The figure shows three views and two pictorial views of one solid part (mm, origin at its lowest corner). Answer the questions. A direction names the side the tool comes from. Give positions to 0.01 mm unless a question says otherwise; leave off trailing zeros. Write each loop counter-clockwise with the first axis right and the second up, starting at its lowest first coordinate (ties: lowest second). Pieces come first, ordered by that corner, then holes. Notation, with made-up numbers: M 44.5,41 L 69.5,41 A30 cw 69.5,63 Z; hole C -16.5,-28 d11. An arc over 180 degrees is marked long. Return JSON: item names as keys, results as strings.
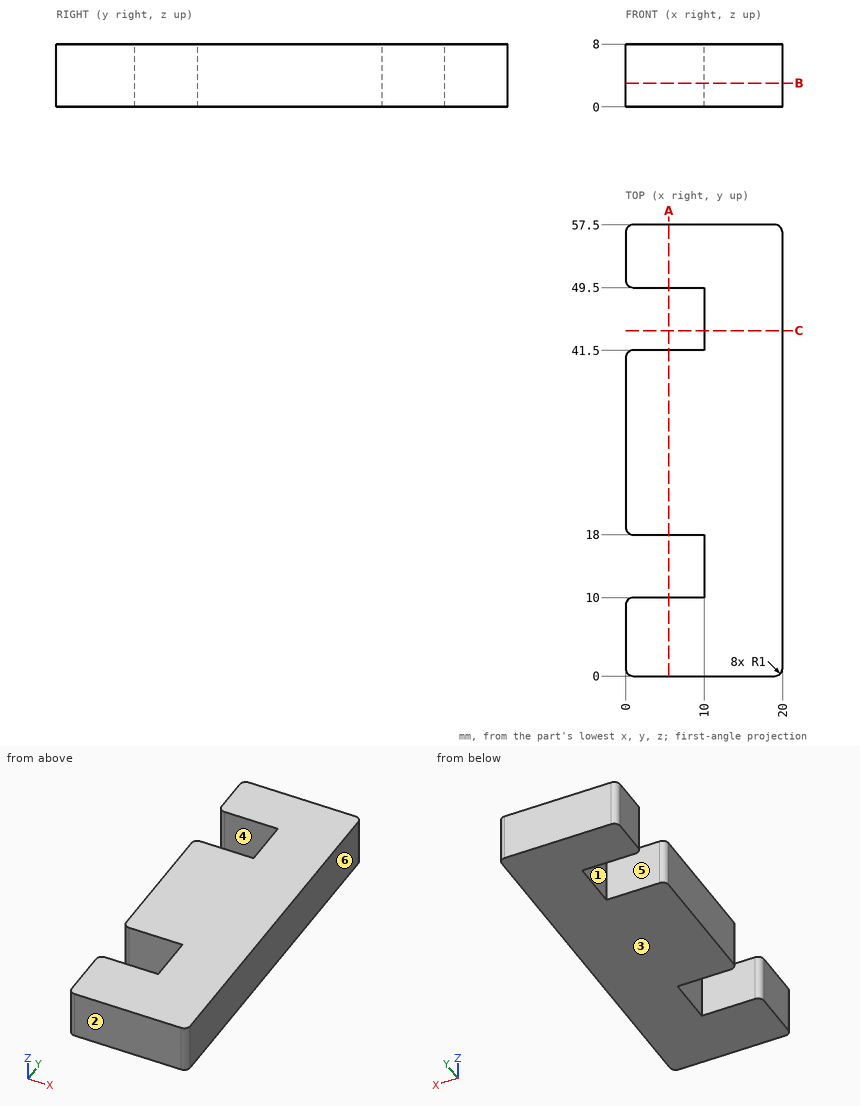
Item 1: Which of the six approach directions +Z, -Z, +X, -X, +Y, -Y give full straight-line access (tool end or side, diameter ignored) to the marked faces 5 and 6?
Geometry results:
{"face 5": "+Z, -Z, -X", "face 6": "+Z, -Z, +X, +Y, -Y"}
Item 2: Find the intervals of material crossed by line 1 (Y direction, x = 8, z = 5.25); line 2 (X direction, y = 45.5, z = 2.5), in increasing order.
Geometry results:
{"line 1": "y = 0 to 10, 18 to 41.5, 49.5 to 57.5", "line 2": "x = 10 to 20"}
Item 3: A cutting plane is placed at A-A, the plane x = 5.5. Write down the section's boundary in (y, z), plus the area to 3 significant figures.
Geometry results:
{"outline": "M 0,0 L 10,0 L 10,8 L 0,8 Z; M 18,0 L 41.5,0 L 41.5,8 L 18,8 Z; M 49.5,0 L 57.5,0 L 57.5,8 L 49.5,8 Z", "area": "332 mm2"}
Item 4: Determine the mould class of the marked faces 1, 2, 3 and 4 for opening direction Y: +Y half, -Y half, draft (parallel to the pull), parting line (faces both ways), or undercut.
Geometry results:
{"face 1": "undercut", "face 2": "-Y half", "face 3": "draft", "face 4": "undercut"}
Item 5: A cutting plane is placed at B-B, the plane z = 3. Write down the section's boundary in (x, y), plus the area to 3 significant figures.
Geometry results:
{"outline": "M 0,1 A1 ccw 1,0 L 19,0 A1 ccw 20,1 L 20,56.5 A1 ccw 19,57.5 L 1,57.5 A1 ccw 0,56.5 L 0,50.5 A1 ccw 1,49.5 L 10,49.5 L 10,41.5 L 1,41.5 A1 ccw 0,40.5 L 0,19 A1 ccw 1,18 L 10,18 L 10,10 L 1,10 A1 ccw 0,9 Z", "area": "988 mm2"}
Item 6: A cutting plane is placed at C-C, the plane y = 44. Write down the section's boundary in (x, z), plus the area to 3 significant figures.
Geometry results:
{"outline": "M 10,0 L 20,0 L 20,8 L 10,8 Z", "area": "80.0 mm2"}
Item 7: Given pin 1 Ø2.5 at (y, z) = (47, 5.5) entering from -X; pin 2 Ø3 at (x, y) = (8, 45) entering from -Z, each flat-ended and moving along its own axis, determine where each tip first touches the part or whether it passes through.
Geometry results:
{"pin 1": "stops at x = 10", "pin 2": "passes through"}
